Read the model definition and answer for the solid it produces. Units are mm, in the model's axes. A direction names the side the tool comes from. Coordinates: 2 decimals unless noted, no trailing zeros. Write each loop counter-clockwise with the first axis right and the second up, starting at its lowest first coordinate (ties: lowest second). Pieces come first, ordered by that corner, then holes. Notation, with made-up numbers: (28.25, -3) -> (83.25, -3) arc R19 cw to (83.25, 26) -> close; hole circle Ø5 at (29, 3). An arc over 180 degrees is marked (long way). Answer in a Markdown table with one row per item. Add a question column.
Item 1: Section C-C on x = 0 is taken. Write down the section's boundary in (y, z).
Item 2: For a pull along X with two mould halves and no side action, classify faces 4 (the face through (83, 22, 1)), 5 (the face through (-84, 0, 1)), 6 (the face through (84.621, 17.336, 1.479)), 7 (the face through (84.5, -17.4, 1.5)) as +X half, -X half, draft (parallel to the pull), parting line (faces both ways), or undercut.
Item 3: Section A-A on x = -79 is taken. Write down the section's boundary in (y, z), then the cut area to 3 significant figures.
Item 4: Given pin 1 Ø1 at (y, z) = (-17, -1.5) entering from +X; pin 2 Ø1.2 at (x, z) = (91, -1) entering from -Y; pin 3 Ø0.5 at (x, z) = (76, -0.5) entering from -Y, each flat-ended and moving along its own axis, determine where each tip first touches the part or whether it passes through.
Item 5: Which of the six approach directions +Z, -Z, +X, -X, +Y, -Y give full straight-line access (tool end or side, diameter ignored) to faces 1 (the face through (-0.16, 11.5, -1.49)), 2 (the face through (-0.1, 13.5, -0.7)), 3 (the face through (83, -22, 1))?
Item 6: Straight lines are drawn through the part: line 1 (Y direction, x = 79, z = 2.4); line 2 (Y direction, x = -79, z = 0.6); line 3 (X direction, y = 19.5, z = -0.3). For each, find the intervals that lie inside material, in ascending order. Write a range as from..to.
Item 7: Section B-B on y = 2 is taken. Write down the section's boundary in (x, z), then the cut area to 3 significant figures.
```python
from build123d import *

# Parameters (mm, degrees)
SKETCH1_R           = 3
BOSS_EXTRUDE1_DEPTH = 3
BOSS_EXTRUDE2_DEPTH = 2
CHAMFER1_SIZE       = 0.5
FILLET1_R           = 1
SKETCH3_R           = 1.6
CUT_EXTRUDE1_DEPTH  = 103.961157725


with BuildPart() as part:
    # Sketch1 → Boss-Extrude1 (new body)
    with BuildSketch(Plane.XY):
        with BuildLine():
            Line((87.658312395, -17.5), (100, -17.5))
            Line((100, -17.5), (100, 17.5))
            Line((100, 17.5), (87.658312395, 17.5))
            ThreePointArc((87.658312395, 17.5), (84.581362835, 17.356617963), (83, 20))
            Line((83, 20), (83, 24))
            Line((83, 24), (-84, 24))
            Line((-84, 24), (-84, -24))
            Line((-84, -24), (83, -24))
            Line((83, -24), (83, -20))
            ThreePointArc((83, -20), (84.581362835, -17.356617963), (87.658312395, -17.5))
        make_face()
        with Locations((-79, -10)):
            Circle(SKETCH1_R, mode=Mode.SUBTRACT)
        with Locations((-79, 10)):
            Circle(SKETCH1_R, mode=Mode.SUBTRACT)
    extrude(amount=BOSS_EXTRUDE1_DEPTH)

    # Sketch2 → Boss-Extrude2 (add)
    with BuildSketch(Plane(origin=(0, 0, 0), x_dir=(-1, 0, 0), z_dir=(0, 0, -1))):
        with BuildLine():
            Line((-73.5, 20), (-73.5, 9.5))
            Line((-73.5, 9.5), (-77.5, 9.5))
            Line((-77.5, 9.5), (-77.5, 15))
            Line((-77.5, 15), (-97.5, 15))
            Line((-97.5, 15), (-97.5, -15))
            Line((-97.5, -15), (-77.5, -15))
            Line((-77.5, -15), (-77.5, -9.5))
            Line((-77.5, -9.5), (-73.5, -9.5))
            Line((-73.5, -9.5), (-73.5, -20))
            ThreePointArc((-73.5, -20), (-73.353553391, -20.353553391), (-73, -20.5))
            Line((-73, -20.5), (-6, -20.5))
            ThreePointArc((-6, -20.5), (-5.646446609, -20.353553391), (-5.5, -20))
            Line((-5.5, -20), (-5.5, -19))
            ThreePointArc((-5.5, -19), (0, -13.5), (5.5, -19))
            Line((5.5, -19), (5.5, -20))
            ThreePointArc((5.5, -20), (5.646446609, -20.353553391), (6, -20.5))
            Line((6, -20.5), (73, -20.5))
            ThreePointArc((73, -20.5), (73.353553391, -20.353553391), (73.5, -20))
            Line((73.5, -20), (73.5, 20))
            ThreePointArc((73.5, 20), (73.353553391, 20.353553391), (73, 20.5))
            Line((73, 20.5), (6, 20.5))
            ThreePointArc((6, 20.5), (5.646446609, 20.353553391), (5.5, 20))
            Line((5.5, 20), (5.5, 19))
            ThreePointArc((5.5, 19), (0, 13.5), (-5.5, 19))
            Line((-5.5, 19), (-5.5, 20))
            ThreePointArc((-5.5, 20), (-5.646446609, 20.353553391), (-6, 20.5))
            Line((-6, 20.5), (-73, 20.5))
            ThreePointArc((-73, 20.5), (-73.353553391, 20.353553391), (-73.5, 20))
        make_face()
        with BuildLine():
            Line((-7.483314774, 18.5), (-71.5, 18.5))
            Line((-71.5, 18.5), (-71.5, 7.5))
            Line((-71.5, 7.5), (-79.5, 7.5))
            Line((-79.5, 7.5), (-79.5, 13))
            Line((-79.5, 13), (-95.5, 13))
            Line((-95.5, 13), (-95.5, -13))
            Line((-95.5, -13), (-79.5, -13))
            Line((-79.5, -13), (-79.5, -7.5))
            Line((-79.5, -7.5), (-71.5, -7.5))
            Line((-71.5, -7.5), (-71.5, -18.5))
            Line((-71.5, -18.5), (-7.483314774, -18.5))
            ThreePointArc((-7.483314774, -18.5), (0, -11.5), (7.483314774, -18.5))
            Line((7.483314774, -18.5), (71.5, -18.5))
            Line((71.5, -18.5), (71.5, 18.5))
            Line((71.5, 18.5), (7.483314774, 18.5))
            ThreePointArc((7.483314774, 18.5), (0, 11.5), (-7.483314774, 18.5))
        make_face(mode=Mode.SUBTRACT)
    extrude(amount=BOSS_EXTRUDE2_DEPTH)

    # Chamfer1
    chamfer1_edges = [part.edges().sort_by_distance(p)[0] for p in [
        (73.353553391, 20.353553391, -2),
        (73.5, 14.75, -2),
        (75.5, 9.5, -2),
        (77.5, 12.25, -2),
        (87.5, 15, -2),
        (97.5, 0, -2),
        (87.5, -15, -2),
        (77.5, -12.25, -2),
        (75.5, -9.5, -2),
        (73.5, -14.75, -2),
        (73.353553391, -20.353553391, -2),
        (39.5, -20.5, -2),
        (5.646446609, -20.353553391, -2),
        (5.5, -19.5, -2),
        (0, -13.5, -2),
        (-5.5, -19.5, -2),
        (-5.646446609, -20.353553391, -2),
        (-39.5, -20.5, -2),
        (-73.353553391, -20.353553391, -2),
        (-73.5, 0, -2),
        (-73.353553391, 20.353553391, -2),
        (-39.5, 20.5, -2),
        (-5.646446609, 20.353553391, -2),
        (-5.5, 19.5, -2),
        (0, 13.5, -2),
        (5.5, 19.5, -2),
        (5.646446609, 20.353553391, -2),
        (39.5, 20.5, -2),
    ]]
    chamfer(chamfer1_edges, length=CHAMFER1_SIZE - 0.0001)  # a hair under: the kernel refuses the full size

    # Fillet1
    fillet1_edges = [part.edges().sort_by_distance(p)[0] for p in [
        (0, 11.5, 0),
        (39.491657387, 18.5, 0),
        (71.5, 13, 0),
        (75.5, 7.5, 0),
        (79.5, 10.25, 0),
        (87.5, 13, 0),
        (95.5, 0, 0),
        (87.5, -13, 0),
        (79.5, -10.25, 0),
        (75.5, -7.5, 0),
        (71.5, -13, 0),
        (39.491657387, -18.5, 0),
        (0, -11.5, 0),
        (-39.491657387, -18.5, 0),
        (-71.5, 0, 0),
        (-39.491657387, 18.5, 0),
    ]]
    fillet(fillet1_edges, radius=FILLET1_R)

    # Sketch3 → Cut-Extrude1 (cut, through all)
    with BuildSketch(Plane.XY.offset(3)):
        with Locations((-79, 19)):
            Circle(SKETCH3_R)
        with Locations((-79, -19)):
            Circle(SKETCH3_R)
        with Locations((79, 19)):
            Circle(SKETCH3_R)
        with Locations((79, -19)):
            Circle(SKETCH3_R)
    extrude(amount=-CUT_EXTRUDE1_DEPTH, mode=Mode.SUBTRACT)


solid = part.part
```
Results below:
| question | item | result |
|---|---|---|
| 1 | outline | (-24, 0) -> (-13.5, 0) -> (-13.5, -1.5) -> (-13, -2) -> (-11.5, -2) -> (-11.5, -1) arc R1 cw to (-10.5, 0) -> (10.5, 0) arc R1 cw to (11.5, -1) -> (11.5, -2) -> (13, -2) -> (13.5, -1.5) -> (13.5, 0) -> (24, 0) -> (24, 3) -> (-24, 3) -> close |
| 2 | face 4 | +X half |
| 2 | face 5 | -X half |
| 2 | face 6 | undercut |
| 2 | face 7 | undercut |
| 3 | outline | (-24, 0) -> (-20.6, 0) -> (-20.6, 3) -> (-24, 3) -> close; (-17.4, 0) -> (-13, 0) -> (-13, 3) -> (-17.4, 3) -> close; (-7, 0) -> (7, 0) -> (7, 3) -> (-7, 3) -> close; (13, 0) -> (17.4, 0) -> (17.4, 3) -> (13, 3) -> close; (20.6, 0) -> (24, 0) -> (24, 3) -> (20.6, 3) -> close |
| 3 | area | 88.8 mm2 |
| 4 | pin 1 | stops at x = 73.5 |
| 4 | pin 2 | stops at y = -15 |
| 4 | pin 3 | stops at y = -9.5 |
| 5 | face 1 | -Z |
| 5 | face 2 | -Z, +Y |
| 5 | face 3 | +Z, -Z, +X, -Y |
| 6 | line 1 | y = -24..-20.6, -17.4..17.4, 20.6..24 |
| 6 | line 2 | y = -24..-20.6, -17.4..-13, -7..7, 13..17.4, 20.6..24 |
| 6 | line 3 | x = -73.5..-5.5, 5.5..73.5 |
| 7 | outline | (-84, 0) -> (-73.5, 0) -> (-73.5, -1.5) -> (-73, -2) -> (-71.5, -2) -> (-71.5, -1) arc R1 cw to (-70.5, 0) -> (94.5, 0) arc R1 cw to (95.5, -1) -> (95.5, -2) -> (97, -2) -> (97.5, -1.5) -> (97.5, 0) -> (100, 0) -> (100, 3) -> (-84, 3) -> close |
| 7 | area | 560 mm2 |
